Read the model definition and answer for the solid it produces. Units are mm, in the model's axes. Face numbers are marked on the shaded views. A direction names the side the tool comes from. Give positions to 0.01 mm unless a question says otherwise; leave off trailing zeros. Order: outer loops, then holes, each group sorted by start corner. A loop starts at its lowest first (then second) coordinate and runs counter-clockwise, first axis right, second up. Notation, with made-up numbers: (38.5, -7) - (88.5, -7) arc R6 ccw to (88.5, 2) - close; hole circle Ø4 at (-6, -12.5). An arc over 180 degrees is marked (long way). Use a Markdown table: item, result. Add a question column.
1. A cutting plane is placed at D-D on y = -3.5. Determine the outline of the cut face in (x, z), and give its area (3 significant figures).
2. Which of the six approach directions +Z, -Z, +X, -X, +Y, -Y give full straight-line access (tool end or side, diameter ignored) to the marked faces 1, 2, 3, 4 and 5?
3. A cutting plane is placed at A-A on y = 3.5. Determine the outline of the cut face in (x, z), and give its area (3 significant figures).
4. Flat-ended cylindrical pins translate along their axes: P1, Ø2, axis at y = 12, z = -3.5, coming from the -X side; P2, Ø1.6, axis at x = 9.5, y = 8.5, coming from the -Z side; P3, Ø2, axis at x = -7.5, y = -2, coming from the -Z side. Find the tip coordinate at first contact, or state that the pin passes through.
5. A cutting plane is placed at B-B on x = 0. Determine the outline of the cut face in (y, z), and give its area (3 significant figures).
6. A cutting plane is placed at C-C on z = 6.25. Determine the outline of the cut face in (x, y), and give its area (3 significant figures).
7. Consider L1, parallel to X at y = 11.5, z = 0.25; L2, parallel to Z at x = 10, y = 11.5; L3, parallel to Y at x = 6.5, z = 7. Determine where each line is inside the solid, lowest interval first.
```python
from build123d import *

# Parameters (mm, degrees)
F0_R     = 7.65
F1_DEPTH = 17
F2_W     = 17
F2_H     = 17
F3_DEPTH = 22
F4_R     = 0.75
F5_DEPTH = 22


# Not quite as in the source:
# - a pattern or mirror of a feature is missing from the dataset's text; its kind, count and spacing are read off the source's solid


with BuildPart() as f1:
    # F0 (on Front) → F1 (new body)
    with BuildSketch(Plane.XZ):
        Circle(F0_R)
    extrude(amount=F1_DEPTH)

    # F2 (on Front) → F3 (join)
    with BuildSketch(Plane.XZ):
        Rectangle(F2_W, F2_H)
    extrude(amount=-F3_DEPTH)

    # F4 (on Front) → F5 (join)
    with BuildSketch(Plane.XZ):
        with BuildLine():
            ThreePointArc((10, -1.5), (11.0606601718, -1.0606601718), (11.5, 0))
            ThreePointArc((11.5, 0), (11.0606601718, 1.0606601718), (10, 1.5))
            ThreePointArc((10, 1.5), (8.9393398282, 1.0606601718), (8.5, 0))
            ThreePointArc((8.5, 0), (8.9393398282, -1.0606601718), (10, -1.5))
        make_face()
        with Locations((10, 0)):
            Circle(F4_R, mode=Mode.SUBTRACT)
        with BuildLine():
            ThreePointArc((8.5, 0), (8.9393398282, 1.0606601718), (10, 1.5))
            Line((10, 1.5), (8.5, 1.5))
            Line((8.5, 1.5), (8.5, 0))
        make_face()
        with BuildLine():
            Line((8.5, -1.5), (10, -1.5))
            ThreePointArc((10, -1.5), (8.9393398282, -1.0606601718), (8.5, 0))
            Line((8.5, 0), (8.5, -1.5))
        make_face()
    f5 = extrude(amount=-F5_DEPTH)

    # F5_copies: F5 across plane
    add(f5.mirror(Plane(origin=(0, 0, 0), x_dir=(0, 0, -1), z_dir=(-1, 0, 0))))


solid = f1.part
```
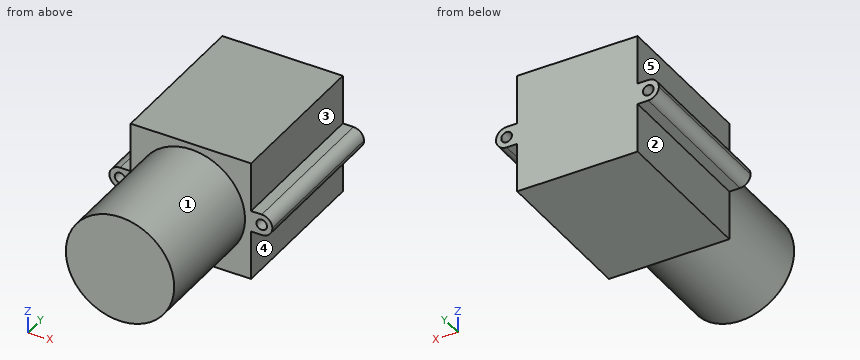
Output values:
| question | item | result |
|---|---|---|
| 1 | outline | circle Ø15.3 at (0, 0) |
| 1 | area | 184 mm² |
| 2 | face 1 | -Y |
| 2 | face 2 | -Z, -X, +Y, -Y |
| 2 | face 3 | +Z, +X, +Y, -Y |
| 2 | face 4 | -Z, +X, +Y, -Y |
| 2 | face 5 | +Z, -X, +Y, -Y |
| 3 | outline | (-10, -1.5) - (-8.5, -1.5) - (-8.5, -8.5) - (8.5, -8.5) - (8.5, -1.5) - (10, -1.5) arc R1.5 ccw to (10, 1.5) - (8.5, 1.5) - (8.5, 8.5) - (-8.5, 8.5) - (-8.5, 1.5) - (-10, 1.5) arc R1.5 ccw to start; hole circle Ø1.5 at (-10, 0); hole circle Ø1.5 at (10, 0) |
| 3 | area | 302 mm² |
| 4 | P1 | x = -8.5 |
| 4 | P2 | z = -1.5 |
| 4 | P3 | z = -4.03 |
| 5 | outline | (-17, -7.65) - (0, -7.65) - (0, -8.5) - (22, -8.5) - (22, 8.5) - (0, 8.5) - (0, 7.65) - (-17, 7.65) - close |
| 5 | area | 634 mm² |
| 6 | outline | (-8.5, 0) - (-4.41, 0) - (-4.41, -17) - (4.41, -17) - (4.41, 0) - (8.5, 0) - (8.5, 22) - (-8.5, 22) - close |
| 6 | area | 524 mm² |
| 7 | L1 | -11.48 to -10.71, -9.29 to 9.29, 10.71 to 11.48 |
| 7 | L2 | -1.5 to -0.75, 0.75 to 1.5 |
| 7 | L3 | 0 to 22 |
